```python
from build123d import *

# Parameters (mm, degrees)
PAD009_DEPTH    = 6
SKETCH051_R     = 1.6
HOLE023_DEPTH   = 25
SKETCH052_R     = 12.5
POCKET005_DEPTH = 6.001
SKETCH057_R     = 1.25
HOLE024_DEPTH   = 25
SKETCH054_R     = 1.25
HOLE025_DEPTH   = 25
SKETCH058_R     = 3.6
HOLE026_DEPTH   = 25
SKETCH056_R     = 2.65
HOLE027_DEPTH   = 25
SKETCH062_R     = 1.6
HOLE031_DEPTH   = 25


with BuildPart() as part:
    # Sketch059 → Pad009 (new body)
    with BuildSketch(Plane.XY):
        with BuildLine():
            Line((-38, 22), (38, 22))
            ThreePointArc((41, 19), (40.12132, 21.12132), (38, 22))
            Line((41, 19), (41, -136))
            ThreePointArc((38, -139), (40.12132, -138.12132), (41, -136))
            Line((38, -139), (-38, -139))
            ThreePointArc((-41, -136), (-40.12132, -138.12132), (-38, -139))
            Line((-41, -136), (-41, 19))
            ThreePointArc((-38, 22), (-40.12132, 21.12132), (-41, 19))
        make_face()
    extrude(amount=PAD009_DEPTH)

    # Sketch051 (on Face10 of Pad009) → Hole023 (cut)
    with BuildSketch(Plane.XY.offset(6)):
        with Locations((-15.5, 15.5)):
            Circle(SKETCH051_R)
        with Locations((15.5, 15.5)):
            Circle(SKETCH051_R)
        with Locations((-15.5, -15.5)):
            Circle(SKETCH051_R)
        with Locations((15.5, -15.5)):
            Circle(SKETCH051_R)
    extrude(amount=-HOLE023_DEPTH, mode=Mode.SUBTRACT)

    # Sketch052 (on Face5 of Hole023) → Pocket005 (cut, through all)
    with BuildSketch(Plane.XY.offset(6)):
        Circle(SKETCH052_R)
    extrude(amount=-POCKET005_DEPTH, mode=Mode.SUBTRACT)

    # Sketch057 (on Face5 of Pocket005) → Hole024 (cut)
    with BuildSketch(Plane.XY.offset(6)):
        with Locations((-13, -53)):
            Circle(SKETCH057_R)
        with Locations((-13, -73)):
            Circle(SKETCH057_R)
        with Locations((-13, -93)):
            Circle(SKETCH057_R)
        with Locations((-13, -113)):
            Circle(SKETCH057_R)
        with Locations((13, -53)):
            Circle(SKETCH057_R)
        with Locations((13, -73)):
            Circle(SKETCH057_R)
        with Locations((13, -93)):
            Circle(SKETCH057_R)
        with Locations((13, -113)):
            Circle(SKETCH057_R)
    extrude(amount=-HOLE024_DEPTH, mode=Mode.SUBTRACT)

    # Sketch054 (on Face5 of Hole024) → Hole025 (cut)
    with BuildSketch(Plane.XY.offset(6)):
        with Locations((0, -129)):
            Circle(SKETCH054_R)
    extrude(amount=-HOLE025_DEPTH, mode=Mode.SUBTRACT)

    # Sketch058 (on Face5 of Hole025) → Hole026 (cut)
    with BuildSketch(Plane.XY.offset(6)):
        with Locations((-31, -47)):
            Circle(SKETCH058_R)
        with Locations((31, -47)):
            Circle(SKETCH058_R)
    extrude(amount=-HOLE026_DEPTH, mode=Mode.SUBTRACT)

    # Sketch056 (on Face5 of Hole026) → Hole027 (cut)
    with BuildSketch(Plane.XY.offset(6)):
        with Locations((-31, -107)):
            Circle(SKETCH056_R)
        with Locations((31, -107)):
            Circle(SKETCH056_R)
    extrude(amount=-HOLE027_DEPTH, mode=Mode.SUBTRACT)

    # Sketch062 (on Face5 of Hole027) → Hole031 (cut)
    with BuildSketch(Plane.XY.offset(6)):
        with Locations((-23.5, -117)):
            Circle(SKETCH062_R)
        with Locations((23.5, -117)):
            Circle(SKETCH062_R)
    extrude(amount=-HOLE031_DEPTH, mode=Mode.SUBTRACT)


with BuildPart() as part_1:
    # Body019 placement: moved
    add(part.part.moved(Location((0, 0, 40))))


solid = part_1.part
```
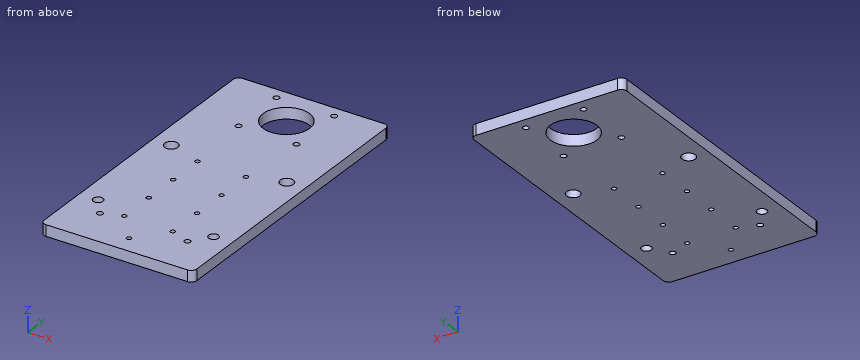
Check sheet for the modelled part. Datum: model origin and axes. Units: mm. Give positions to 0.01 mm unless a question says otherwise; leave off trailing zeros. Write each loop counter-clockwise with the first axis right and the second up, starting at its lowest first coordinate (ties: lowest second). Pieces come first, ordered by that corner, then holes. Notation, with made-up numbers: (51, 79) - (74, 79) arc R21 cw to (74, 98) - close; hole circle Ø10 at (50, -2). An arc over 180 degrees is marked (long way). Answer as a JSON object with one key per item and string values. Group by question number.
1) Sectioned sample at D-D (x = 23.5). Record the cut outline in (y, z).
2) Sectioned sample at B-B (z = 44.65). Give the number of separate pieces and of enclosed holes in the cut face, then the cut area to 3 significant figures.
3) Sectioned sample at A-A (x = -31). Record the cut outline in (y, z), then the cut area to 3 significant figures.
4) Sectioned sample at C-C (y = 15.5). Record the cut outline in (x, z).
5) Depth check by flat-ended pin: P1, Ø3, axis at x = -13, y = -113, coming from the +Z side. Enter the tip coordinate at first touch or a pass-through.
6) Thickness scan on probe 1 along X at (y, z) = (-117, 41.8); probe 2 along Y at (x, z) = (31, 42.75); probe 3 along X at (y, z) = (-113, 43). Record the ranges inside material, lowest first. Write a range as from..to.
Geometry results:
{
 "1": {"outline": "(-139, 40) - (-118.6, 40) - (-118.6, 46) - (-139, 46) - close; (-115.4, 40) - (22, 40) - (22, 46) - (-115.4, 46) - close"},
 "2": {"separate pieces": "1", "enclosed holes": "20", "area": "12,500 mm^2"},
 "3": {"outline": "(-139, 40) - (-109.65, 40) - (-109.65, 46) - (-139, 46) - close; (-104.35, 40) - (-50.6, 40) - (-50.6, 46) - (-104.35, 46) - close; (-43.4, 40) - (22, 40) - (22, 46) - (-43.4, 46) - close", "area": "891 mm^2"},
 "4": {"outline": "(-41, 40) - (-17.1, 40) - (-17.1, 46) - (-41, 46) - close; (-13.9, 40) - (13.9, 40) - (13.9, 46) - (-13.9, 46) - close; (17.1, 40) - (41, 40) - (41, 46) - (17.1, 46) - close"},
 "5": {"P1": "stops at z = 46"},
 "6": {"probe 1": "x = -41..-25.1, -21.9..21.9, 25.1..41", "probe 2": "y = -139..-109.65, -104.35..-50.6, -43.4..22", "probe 3": "x = -41..-14.25, -11.75..11.75, 14.25..41"}
}
